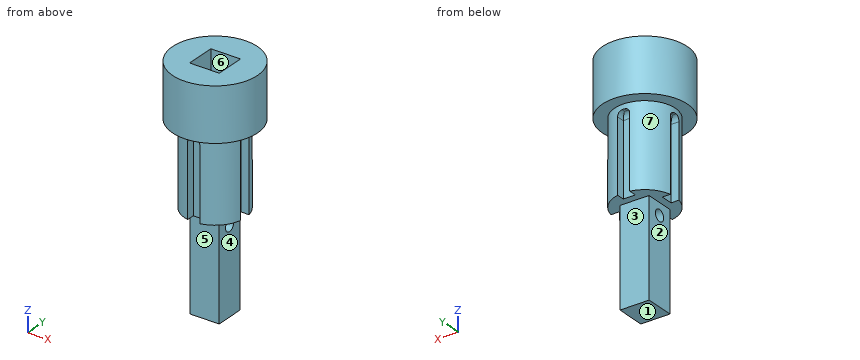
from build123d import *

# Parameters (mm, degrees)
ESBO_O1_R                  = 17.5
RESSALTO_EXTRUS_O1_DEPTH   = 22
ESBO_O2_W                  = 12.25
ESBO_O2_H                  = 12.25
CORTE_EXTRUS_O1_DEPTH      = 25
ESBO_O3_R                  = 12.5
RESSALTO_EXTRUS_O2_DEPTH   = 34
ESBO_O4_W                  = 5
ESBO_O4_H                  = 6
ESBO_O4_W_2                = 6
ESBO_O4_H_2                = 5
CORTE_EXTRUS_O2_DEPTH      = 32
FILETE2_R                  = 2
FILETE3_R                  = 2
FILETE4_R                  = 2
FILETE5_R                  = 2
ESBO_O5_W                  = 12
ESBO_O5_H                  = 12
RESSALTO_EXTRUS_O3_DEPTH   = 40
CORTE_EXTRUS_O3_DEPTH      = 14
CORTE_EXTRUS_O3_DEPTH_BACK = 15
ESBO_O6_R                  = 2.35


with BuildPart() as part:
    # Esboço1 → Ressalto-extrusão1 (new body)
    with BuildSketch(Plane.XY):
        Circle(ESBO_O1_R)
    extrude(amount=RESSALTO_EXTRUS_O1_DEPTH)

    # Esboço2 → Corte-extrusão1 (cut)
    with BuildSketch(Plane(origin=(0, 0, 0), x_dir=(-1, 0, 0), z_dir=(0, 0, -1))):
        Rectangle(ESBO_O2_W, ESBO_O2_H)
    extrude(amount=-CORTE_EXTRUS_O1_DEPTH, mode=Mode.SUBTRACT)

    # Esboço3 → Ressalto-extrusão2 (add)
    with BuildSketch(Plane(origin=(0, 0, 0), x_dir=(-1, 0, 0), z_dir=(0, 0, -1))):
        with Locations(Location((0, 0, 0), (0, 0, 180))):
            Circle(ESBO_O3_R)
    extrude(amount=RESSALTO_EXTRUS_O2_DEPTH)

    # Esboço4 → Corte-extrusão2 (cut)
    with BuildSketch(Plane(origin=(0, 0, -34), x_dir=(-1, 0, 0), z_dir=(0, 0, -1))):
        with Locations((0, -12)):
            Rectangle(ESBO_O4_W, ESBO_O4_H)
        with Locations((0, 12)):
            Rectangle(ESBO_O4_W, ESBO_O4_H)
        with Locations((12, 0)):
            Rectangle(ESBO_O4_W_2, ESBO_O4_H_2)
        with Locations((-12, 0)):
            Rectangle(ESBO_O4_W_2, ESBO_O4_H_2)
    extrude(amount=-CORTE_EXTRUS_O2_DEPTH, mode=Mode.SUBTRACT)

    # Filete2
    filete2_edges = [part.edges().sort_by_distance(p)[0] for p in [
        (10.623724357, 2.5, -2),
        (10.623724357, -2.5, -2),
        (9, 0, -2),
    ]]
    fillet(filete2_edges, radius=FILETE2_R)

    # Filete3
    filete3_edges = [part.edges().sort_by_distance(p)[0] for p in [
        (2.5, -10.623724357, -2),
        (-2.5, -10.623724357, -2),
        (0, -9, -2),
    ]]
    fillet(filete3_edges, radius=FILETE3_R)

    # Filete4
    filete4_edges = [part.edges().sort_by_distance(p)[0] for p in [
        (-10.623724357, 2.5, -2),
        (-10.623724357, -2.5, -2),
        (-9, 0, -2),
    ]]
    fillet(filete4_edges, radius=FILETE4_R)

    # Filete5
    filete5_edges = [part.edges().sort_by_distance(p)[0] for p in [
        (2.5, 10.623724357, -2),
        (-2.5, 10.623724357, -2),
        (0, 9, -2),
    ]]
    fillet(filete5_edges, radius=FILETE5_R)

    # Esboço5 → Ressalto-extrusão3 (add)
    with BuildSketch(Plane(origin=(0, 0, -34), x_dir=(-1, 0, 0), z_dir=(0, 0, -1))):
        Rectangle(ESBO_O5_W, ESBO_O5_H)
    extrude(amount=RESSALTO_EXTRUS_O3_DEPTH)

    # Esboço6 → Corte-extrusão3 (cut, two sides: drawn at the far end of the back side and taken through both)
    with BuildSketch(Plane(origin=(6, 0, 0), x_dir=(0, 0, -1), z_dir=(1, 0, 0)).offset(-CORTE_EXTRUS_O3_DEPTH_BACK)):
        with Locations(Location((39, 0, 0), (0, 0, 270))):
            Circle(ESBO_O6_R)
    extrude(amount=CORTE_EXTRUS_O3_DEPTH + CORTE_EXTRUS_O3_DEPTH_BACK, mode=Mode.SUBTRACT)


solid = part.part
Check sheet for the modelled part. Datum: model origin and axes. Units: mm. Face numbers are marked on the shaded views. A direction names the side the tool comes from. Round coordinates to 2 decimals unless told otherwise and drop trailing zeros. Order: outer loops, then holes, each group sorted by start corner. A loop starts at its lowest first (then second) coordinate and runs counter-clockwise, first axis right, second up. Notation, with made-up numbers: M 77,28 L 81,28 A25 ccw 81,44 Z; hole C 6,25.5 d7. An arc over 180 degrees is marked long. One line per item, written item: value. Start each with the question number.
1. Section check C-C on z = 5.5. Enter the section's corners in (x, y) (3 decimals).
2. Section check D-D on y = 14. Enter the section's corners in (x, z), and give its area (3 significant figures).
3. Release check for a two-part mould opening along Y. For the marked faces 4, 5, 6 and 7 record: released by +Y, released by -Y, zero draft, split by the parting line, or undercut.
4. Gauge pin test, flat ends, axial feed: P1, Ø1.6, axis at x = -10.5, z = -14.5, coming from the +Y side; P2, Ø3.5, axis at x = 2.5, y = 2.5, coming from the +Z side; P3, Ø12, axis at y = -11.5, z = 6, coming from the +X side. Record the tip position at first contact, or that the pin passes through.
5. Scan lines: line 1 along Z through (x, y) = (-2, 0); line 2 along Z through (x, y) = (9, -13); line 3 along Z through (x, y) = (-0.5, 12). Record each from-to range of solid material in increasing order.
6. Section check A-A on z = -39. Enter the section's corners in (x, y).
7. Access from +Z, -Z, +X, -X, +Y, -Y to the whole of each face (thin tool, end or side, straight path). Record for the marked faces 1, 2 and 3.
Results found:
1. outline: C 0,0 d35; hole M -6.125,-6.125 L 6.125,-6.125 L 6.125,6.125 L -6.125,6.125 Z
2. outline: M -10.5,0 L 10.5,0 L 10.5,22 L -10.5,22 Z
2. area: 462 mm^2
3. face 4: zero draft
3. face 5: released by -Y
3. face 6: undercut
3. face 7: split by the parting line
4. P1: y = 7.88
4. P2: z = 0
4. P3: x = 16.61
5. line 1: -74 to -41.35, -36.65 to 0
5. line 2: 0 to 22
5. line 3: -2 to 22
6. outline: M -6,-6 L 6,-6 L 6,-2.35 L -6,-2.35 Z; M -6,2.35 L 6,2.35 L 6,6 L -6,6 Z
7. face 1: -Z, +X, -X, +Y, -Y
7. face 2: -Z, -X, +Y, -Y
7. face 3: -Z, +X, -X, +Y
